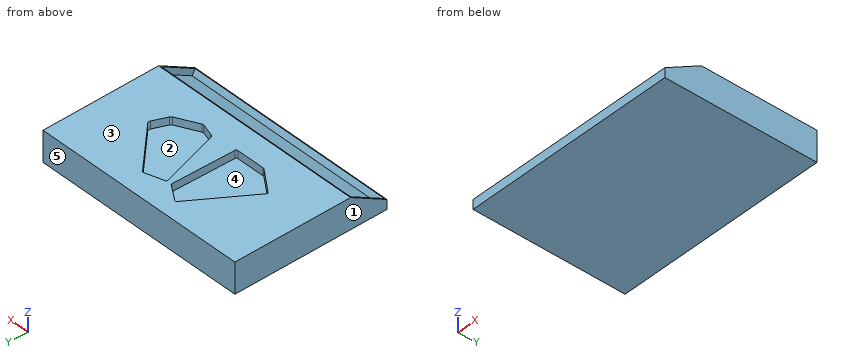
```python
from build123d import *

# Parameters (mm, degrees)
F0_W     = 70
F0_H     = 50
F1_DEPTH = 10
F2_SIZE2 = 6.9282032303
F2_SIZE  = 12
F4_DEPTH = 2.5
F5_W     = 69
F5_H     = 12.8564064606
F6_DEPTH = 2


with BuildPart() as f1:
    # F0 (on Top) → F1 (new body)
    with BuildSketch(Plane.XY):
        with Locations((5.1442100421, 5.2647431195)):
            Rectangle(F0_W, F0_H)
    extrude(amount=F1_DEPTH)

    # F2
    f2_edges = [f1.edges().sort_by_distance(p)[0] for p in [
        (5.14421, -19.735257, 10),
    ]]
    f2_side = f1.faces().sort_by_distance((5.14421, 5.264743, 10))[0]
    chamfer(f2_edges, length=F2_SIZE, length2=F2_SIZE2, reference=f2_side)

    # F3 (on face) → F4 (cut)
    with BuildSketch(Plane.XY.offset(10)):
        with BuildLine():
            ThreePointArc((-1.969263475, 24.8949940758), (-2.3442214304, 24.9714998994), (-2.66345453, 24.7604623731))
            Line((-2.66345453, 24.7604623731), (-14.9844594162, 6.5159764986))
            ThreePointArc((-14.9844594162, 6.5159764986), (-15.0623736344, 6.1485983412), (-14.8625708975, 5.830610602))
            Line((-14.8625708975, 5.830610602), (-7.4070282086, 0.4536706786))
            ThreePointArc((-7.4070282086, 0.4536706786), (-7.1294320931, 0.3131464505), (-6.8220824883, 0.2647431195))
            Line((-6.8220824883, 0.2647431195), (2.3681526499, 0.2647431195))
            ThreePointArc((2.3681526499, 0.2647431195), (2.7169388104, 0.4064859293), (2.8679732491, 0.7513502623))
            Line((2.8679732491, 0.7513502623), (3.410086475, 20.9829822828))
            ThreePointArc((3.410086475, 20.9829822828), (3.3549084959, 21.2250516372), (3.190095552, 21.4107365189))
            Line((3.190095552, 21.4107365189), (-1.969263475, 24.8949940758))
        make_face()
        with BuildLine():
            ThreePointArc((11.8286107336, 23.0692653505), (11.5949478981, 23.2051710927), (11.3246932103, 23.1995947829))
            Line((11.3246932103, 23.1995947829), (5.3912275031, 21.4008405723))
            ThreePointArc((5.3912275031, 21.4008405723), (5.0965360899, 21.1602954599), (5.0563803582, 20.7820197704))
            Line((5.0563803582, 20.7820197704), (10.6604367749, 1.6164084942))
            ThreePointArc((10.6604367749, 1.6164084942), (10.9073063674, 1.195834103), (11.3237327707, 0.9420301136))
            Line((11.3237327707, 0.9420301136), (15.2026586897, -0.2622863149))
            ThreePointArc((15.2026586897, -0.2622863149), (15.579956303, -0.3039895341), (15.9456136146, -0.2020710473))
            Line((15.9456136146, -0.2020710473), (22.8627626989, 3.249037371))
            ThreePointArc((22.8627626989, 3.249037371), (23.1443824723, 3.4583377212), (23.3363661018, 3.7520358986))
            Line((23.3363661018, 3.7520358986), (25.2827025924, 8.3223486347))
            ThreePointArc((25.2827025924, 8.3223486347), (25.3458081315, 8.896965521), (25.0803776052, 9.4104959591))
            Line((25.0803776052, 9.4104959591), (11.8286107336, 23.0692653505))
        make_face()
    extrude(amount=-F4_DEPTH, mode=Mode.SUBTRACT)

    # F5 (on face) → F6 (cut)
    with BuildSketch(Plane(origin=(0, -6.2639412391, 10.8494644817), x_dir=(1, 0, 0), z_dir=(0, -0.5, 0.8660254038))):
        with Locations((5.1442100421, -8.6271321936)):
            Rectangle(F5_W, F5_H)
    extrude(amount=-F6_DEPTH, mode=Mode.SUBTRACT)


solid = f1.part
```
Geometry: final body of the model. Coordinates: model frame, mm. Face numbers are marked on the shaded views. A direction names the side the tool comes from. Round coordinates to 2 decimals unless told otherwise and drop trailing zeros. Loops run counter-clockwise (first coordinate to the right, second up) from the corner with the lowest first, then second, coordinate; pieces in that order, holes last.
Item 1: Line query: L1, parallel to X at y = 13, z = 8.25; L2, parallel to X at y = 20.5, z = 9.5; L3, parallel to Y at x = 36.5, z = 3.5. Output: solid intervals per line, ascending.
Checked values:
L1: x = -29.86 to -10.61, 3.2 to 7.33, 21.6 to 40.14
L2: x = -29.86 to -5.54, 3.4 to 5.14, 14.32 to 40.14
L3: y = -14.99 to 30.26
Item 2: Section B-B, the plane y = 16. Output: boundary loops of the cut face in (x, z), plus the area to 3 significant figures.
Checked values:
outline: (-29.86, 0) - (40.14, 0) - (40.14, 10) - (18.69, 10) - (18.69, 7.5) - (6.45, 7.5) - (6.45, 10) - (3.28, 10) - (3.28, 7.5) - (-8.58, 7.5) - (-8.58, 10) - (-29.86, 10) - close
area: 640 mm2
Item 3: Section C-C, the plane z = 9. State how many separate pieces and enclosed holes the cut face has, plus the area to 3 significant figures.
Checked values:
separate pieces: 1
enclosed holes: 2
area: 2,080 mm2
Item 4: Section D-D, the plane z = 4.75. Output: boundary loops of the cut face in (x, y).
Checked values:
outline: (-29.86, -16.83) - (-29.36, -16.83) - (-29.36, -12.83) - (39.64, -12.83) - (39.64, -16.83) - (40.14, -16.83) - (40.14, 30.26) - (-29.86, 30.26) - close
Item 5: Contact query for a flat-ended pin moving along its axis: P1, Ø1, axis at x = -14.5, y = 16.5, coming from the -Z side. Output: stop coordinate, or through.
Checked values:
P1: stops at z = 0
Item 6: Mould query, pull axis Y, two halves, no side actions, for the marked faces 3, 4 and 5. Classes: released by +Y, released by -Y, zero draft, split by the parting line, or undercut.
Checked values:
face 3: zero draft
face 4: undercut
face 5: released by +Y
Item 7: Section A-A, the plane x = 34. Output: boundary loops of the cut face in (y, z), plus the area to 3 significant figures.
Checked values:
outline: (-19.74, 0) - (30.26, 0) - (30.26, 10) - (-7.74, 10) - (-8.17, 9.75) - (-7.17, 8.02) - (-18.3, 1.59) - (-19.3, 3.32) - (-19.74, 3.07) - close
area: 433 mm2
Item 8: Reachability of the marked faces 1 and 2 from +Z, -Z, +X, -X, +Y, -Y: full face, straight path, thin tool, end or side. Return the list, or none.
Checked values:
face 1: +Z, -Z, -X, +Y, -Y
face 2: +Z
